The model under review builds one solid part; all positions refer to its coordinate system, in mm. A direction names the side the tool comes from. Round coordinates to 2 decimals unless told otherwise and drop trailing zeros. Order: outer loops, then holes, each group sorted by start corner. A loop starts at its lowest first (then second) coordinate and runs counter-clockwise, first axis right, second up.
1) Consider section C-C (y = 4.25). Give the number of separate pieces and of enclosed holes in the cut face, then the cut area to 3 significant figures.
2) Mouldability with a two-part tool opening along Z and no side actions: class faces 1 (the face through (-46.81, 4.83, 18.41)), 2 (the face through (26.93, 4.57, 12.67)), 3 (the face through (-7, 9.525, -39)) as pulls with the +Z half, pulls with the -Z half, needs draft (parallel to the pull), parting line crosses it, or undercut.
3) Machinability: for faces 4 (the face through (23.1, 4.7, -37.5)), 5 (the face through (-7, 0, -39)), which of the approach directions +Z, -Z, +X, -X, +Y, -Y give a long, thin tool a straight path to every point of the face, cutting with its end or side? Answer none if there is none.
4) To check wall thickness, follow L1, parallel to X at y = 7.75, z = -18.5; L2, parallel to Z at x = -41.5, y = 8.75; L3, parallel to X at y = 3.5, z = 13. State the ranges of each line that lie inside material, in increasing order.
5) Consider section B-B (z = -9). Give the boundary of the cut face in (x, y) (3 decimals), then the cut area to 3 significant figures.
6) Clearance check with flat-ended pins moving along their axes: P1, Ø4, axis at x = -41.37, z = -44.14, coming from the -Y side; P2, Ø3, axis at x = 28.48, z = 13.01, coming from the +Y side. State where each tip first meets the part, or that it passes through.
7) Consider section A-A (x = -7). Give the boundary of the cut face in (y, z) (3 decimals), then the cut area to 3 significant figures.
from build123d import *

# Parameters (mm, degrees)
SKETCH1_W           = 82.55
SKETCH1_H           = 69.85
BOSS_EXTRUDE1_DEPTH = 9.525
SKETCH2_W           = 30.48
SKETCH2_H           = 22.86
CUT_EXTRUDE1_DEPTH  = 71.120815038
SKETCH5_R           = 1.5875
CUT_EXTRUDE2_DEPTH  = 71.120815038
FILLET1_R           = 3.175
CHAMFER1_SIZE       = 0.508


with BuildPart() as part:
    # Sketch1 → Boss-Extrude1 (new body)
    with BuildSketch(Plane(origin=(0, 0, 0), x_dir=(1, 0, 0), z_dir=(0, 1, 0))):
        with Locations((-6.44460094, 15.563045741)):
            Rectangle(SKETCH1_W, SKETCH1_H)
    extrude(amount=BOSS_EXTRUDE1_DEPTH)

    # Sketch2 → Cut-Extrude1 (cut, through all)
    with BuildSketch(Plane(origin=(0, 9.525, 0), x_dir=(1, 0, 0), z_dir=(0, 1, 0))):
        with Locations((-21.68460094, 26.993045741)):
            Rectangle(SKETCH2_W, SKETCH2_H)
        with Locations((8.79539906, 26.993045741)):
            Rectangle(SKETCH2_W, SKETCH2_H)
        with Locations((8.79539906, 4.133045741)):
            Rectangle(SKETCH2_W, SKETCH2_H)
        with Locations((-21.68460094, 4.133045741)):
            Rectangle(SKETCH2_W, SKETCH2_H)
    extrude(amount=-CUT_EXTRUDE1_DEPTH, mode=Mode.SUBTRACT)

    # Sketch5 → Cut-Extrude2 (cut, through all)
    with BuildSketch(Plane(origin=(0, 9.525, 0), x_dir=(1, 0, 0), z_dir=(0, 1, 0))):
        with Locations(Location((-41.36960094, 44.138045741, 0), (0, 0, 270))):
            Circle(SKETCH5_R)
        with Locations(Location((28.48039906, 44.138045741, 0), (0, 0, 270))):
            Circle(SKETCH5_R)
        with Locations(Location((28.48039906, -13.011954259, 0), (0, 0, 270))):
            Circle(SKETCH5_R)
        with Locations(Location((-41.36960094, -13.011954259, 0), (0, 0, 270))):
            Circle(SKETCH5_R)
    extrude(amount=-CUT_EXTRUDE2_DEPTH, mode=Mode.SUBTRACT)

    # Fillet1
    fillet1_edges = [part.edges().sort_by_distance(p)[0] for p in [
        (24.03539906, 4.7625, 7.296954259),
        (-36.92460094, 4.7625, 7.296954259),
        (-36.92460094, 4.7625, -38.423045741),
        (24.03539906, 4.7625, -38.423045741),
        (-47.71960094, 4.7625, -50.488045741),
        (34.83039906, 4.7625, -50.488045741),
        (34.83039906, 4.7625, 19.361954259),
        (-47.71960094, 4.7625, 19.361954259),
    ]]
    fillet(fillet1_edges, radius=FILLET1_R)

    # Chamfer1
    chamfer1_edges = [part.edges().sort_by_distance(p)[0] for p in [
        (-41.36960094, 9.525, 11.424454259),
        (28.48039906, 9.525, 11.424454259),
        (28.48039906, 9.525, -45.725545741),
        (-41.36960094, 9.525, -45.725545741),
    ]]
    chamfer(chamfer1_edges, length=CHAMFER1_SIZE)


solid = part.part
Answer below:
1. separate pieces: 1
1. enclosed holes: 5
1. area: 2,950 mm2
2. face 1: pulls with the +Z half
2. face 2: undercut
2. face 3: needs draft
3. face 4: +Y, -Y
3. face 5: +Z, -Z, +X, -X, -Y
4. L1: x = -47.72 to -36.92, 24.04 to 34.83
4. L2: z = -50.49 to -45.72, -42.56 to 11.43, 14.59 to 19.36
4. L3: x = -47.72 to -42.96, -39.78 to 26.89, 30.07 to 34.83
5. outline: (-47.72, 0) - (-36.925, 0) - (-36.925, 9.525) - (-47.72, 9.525) - close; (24.035, 0) - (34.83, 0) - (34.83, 9.525) - (24.035, 9.525) - close
5. area: 206 mm2
6. P1: stops at y = 0
6. P2: passes through
7. outline: (0, -50.488) - (9.525, -50.488) - (9.525, -38.423) - (0, -38.423) - close; (0, 7.297) - (9.525, 7.297) - (9.525, 19.362) - (0, 19.362) - close
7. area: 230 mm2
